Autodesk Inventor part; units mm, degrees
ref_plane "YZ Plane" through (0, 0, 0) normal (1, 0, 0) x (0, 1, 0)
ref_plane "XZ Plane" through (0, 0, 0) normal (0, 1, 0) x (-1, 0, 0)
ref_plane "XY Plane" through (0, 0, 0) normal (0, 0, 1) x (1, 0, 0)
sketch "Эскиз1" plane through (0, 0, 0) normal (0, 0, 1) x (1, 0, 0)
  circle A0 centre (0, 0) radius 6.6
  circle A1 centre (0, 0) radius 10.6
  dimension "d0" = 13.2
  dimension "d1" = 4
extrude "Выдавливание1" add sketch "Эскиз1" along normal blind 7 and the other way blind 12
fillet "Сопряжение1" radius 2 2 edges at (-10.6, 0, 7) (-10.6, 0, -12)
chamfer "Фаска1" distance 1 angle 45 1 edges at (-6.6, 0, -12)
ref_plane "РабПлоскость1" through (0, 0, 0) normal (0, 0, 1) x (1, 0, 0)
sketch "Эскиз2" plane through (0, 0, 0) normal (0, 0, 1) x (1, 0, 0)
  circle A0 centre (0, 0) radius 4
  circle A1 centre (0, 0) radius 8.6
  circle A2 centre (0, 0) radius 7.5
  dimension "d10" = 8
  dimension "d11" = 15
extrude "Выдавливание2" add sketch "Эскиз2" along normal blind 7 contours A2
chamfer "Фаска2" distance 2.5 angle 45 1 edges at (-4, 0, 7)
properties part number "ПодпорныйКаток"
Input: part model. Units: mm. Frame: model coordinates. A direction names the side the tool comes from. Coordinates: 2 decimals unless noted, no trailing zeros. Order: outer loops, then holes, each group sorted by start corner. A loop starts at its lowest first (then second) coordinate and runs counter-clockwise, first axis right, second up. Notation, with made-up numbers: (39, 36) - (46, 36) arc R18 cw to (46, 62) - close; hole circle Ø1 at (71.25, 37). An arc over 180 degrees is marked (long way). Return JSON: item names as keys, results as strings.
Q1. Ray query, probe 1 along Y at (x, z) = (0, -7.5); probe 2 along Y at (x, z) = (0, 1.1); probe 3 along X at (y, z) = (5, -7.5). Return the intervals inside material, ascending.
The answers:
{"probe 1": "y = -10.6 to -6.6, 6.6 to 10.6", "probe 2": "y = -10.6 to -4, 4 to 10.6", "probe 3": "x = -9.35 to -4.31, 4.31 to 9.35"}
Q2. Cut plane C-C (z = -7.25). Return loops of the section in (x, y).
The answers:
{"outline": "circle Ø21.2 at (0, 0); hole circle Ø13.2 at (0, 0)"}
Q3. Access query for faces 5 (the cylindrical face through (-0.867, 3.905, 2.218)), 6 (the flat face through (3, -3, 0)). Directions: +Z, -Z, +X, -X, +Y, -Y. A direction counts if a zero-diameter tool reaches every point of the face in a straight line with its end or side. Return the directions, or none.
The answers:
{"face 5": "+Z, -Z", "face 6": "-Z"}
Q4. Cut plane D-D (z = 1.75). Return loops of the section in (x, y).
The answers:
{"outline": "circle Ø21.2 at (0, 0); hole circle Ø8 at (0, 0)"}
Q5. Cut plane A-A (y = 0). Return loops of the section in (x, z).
The answers:
{"outline": "(-10.6, -10) arc R2 ccw to (-8.6, -12) - (-7.6, -12) - (-6.6, -11) - (-6.6, 0) - (-4, 0) - (-4, 4.5) - (-6.5, 7) - (-8.6, 7) arc R2 ccw to (-10.6, 5) - close; (4, 0) - (6.6, 0) - (6.6, -11) - (7.6, -12) - (8.6, -12) arc R2 ccw to (10.6, -10) - (10.6, 5) arc R2 ccw to (8.6, 7) - (6.5, 7) - (4, 4.5) - close"}
Q6. Draft query along Y for faces 1 (the conical face through (-0.541, 4.121, 4.656)), 2 (the cylindrical face through (9.79, 4.06, -2.61)), 3 (the cylindrical face through (-4.864, 4.461, -5.423)), 4 (the flat face through (0, -8, -12)). Return one class per face: +Y half, -Y half, draft (parallel to the pull), parting line (faces both ways), or undercut.
The answers:
{"face 1": "undercut", "face 2": "parting line", "face 3": "undercut", "face 4": "draft"}
Q7. First-contact query: pin 1 (5 mm diameter, centred on y = -3, z = -2.5, fed in from +X); pin 2 (5 mm diameter, centred on y = 4, z = -4, fed in from +X); pin 3 (9 mm diameter, centred on x = 0, y = 0, fed in from +Z). Flat tips, straight axial feed; report the tip coordinate or a pass-through.
The answers:
{"pin 1": "stops at x = 10.59", "pin 2": "stops at x = 10.49", "pin 3": "stops at z = 5"}
